from build123d import *

# Parameters (mm, degrees)
F1_DEPTH = 25.4
F3_DEPTH = 25.4


with BuildPart() as f1:
    # F0 (on Front) → F1 (new body)
    with BuildSketch(Plane.XZ):
        with BuildLine():
            Line((0, 38.1), (0, 0))
            Line((0, 0), (50.8, 0))
            Line((50.8, 0), (50.8, 38.1))
            ThreePointArc((50.8, 38.1), (47.080256, 47.080256), (38.1, 50.8))
            Line((38.1, 50.8), (12.7, 50.8))
            ThreePointArc((12.7, 50.8), (3.719744, 47.080256), (0, 38.1))
        make_face()
    extrude(amount=F1_DEPTH)

    # F2 (on Front) → F3 (join)
    with BuildSketch(Plane.XZ):
        Polygon((17.737616, 7.724446), (17.737616, 0), (39.861955, 0), (39.861955, 7.724446), (30.707058, 7.724446), (30.707058, 12.492622), (23.459429, 12.492622), (23.459429, 7.724446), align=None)
    extrude(amount=F3_DEPTH)


solid = f1.part
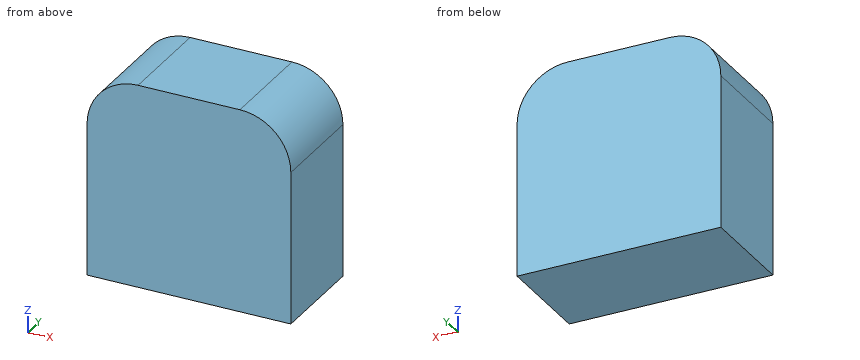
For this review, take the finished solid that the model builds, in its own axes (mm). Coordinates: 2 decimals unless noted, no trailing zeros. Order: outer loops, then holes, each group sorted by start corner. A loop starts at its lowest first (then second) coordinate and runs counter-clockwise, first axis right, second up. Notation, with made-up numbers: (-33.75, 73.5) -> (11.25, 73.5) arc R14 ccw to (11.25, 86.5) -> close; hole circle Ø6 at (86.5, 13.25). An arc over 180 degrees is marked (long way). Return JSON: item names as keys, results as strings.
1. For pin 1 Ø8 at (y, z) = (-13, 43) entering from +X, flat-tipped, find the tip position at first contact; note if it passes through.
Answer block:
{"pin 1": "x = 50.77"}
2. For line 1 (Z direction, x = 12.5, y = -12.25); line 2 (Z direction, x = 46, y = -17.5); line 3 (X direction, y = -10, z = 46), list the stretches that pass through material, from the lowest coordinate up. Write a range as from..to.
Answer block:
{"line 1": "0..50.8", "line 2": "0..48.04", "line 3": "2.76..48.04"}
3. We need section A-A on y = -17. Write out the cut boundary in (x, z).
Answer block:
{"outline": "(0, 0) -> (50.8, 0) -> (50.8, 38.1) arc R12.7 ccw to (38.1, 50.8) -> (12.7, 50.8) arc R12.7 ccw to (0, 38.1) -> close"}
4. We need section B-B on x = 43. Write out the cut boundary in (y, z), and give its area (3 significant figures).
Answer block:
{"outline": "(-25.4, 0) -> (0, 0) -> (0, 49.82) -> (-25.4, 49.82) -> close", "area": "1,270 mm²"}
